Check sheet for the drawn part. Datum: minimum x, y, z corner. Units: mm. A direction names the side the tool comes from. Give positions to 0.01 mm unless a question says otherwise; leave off trailing zeros. Order: outer loops, then holes, each group sorted by start corner. A loop starts at its lowest first (then second) coordinate and runs counter-clockwise, first axis right, second up.
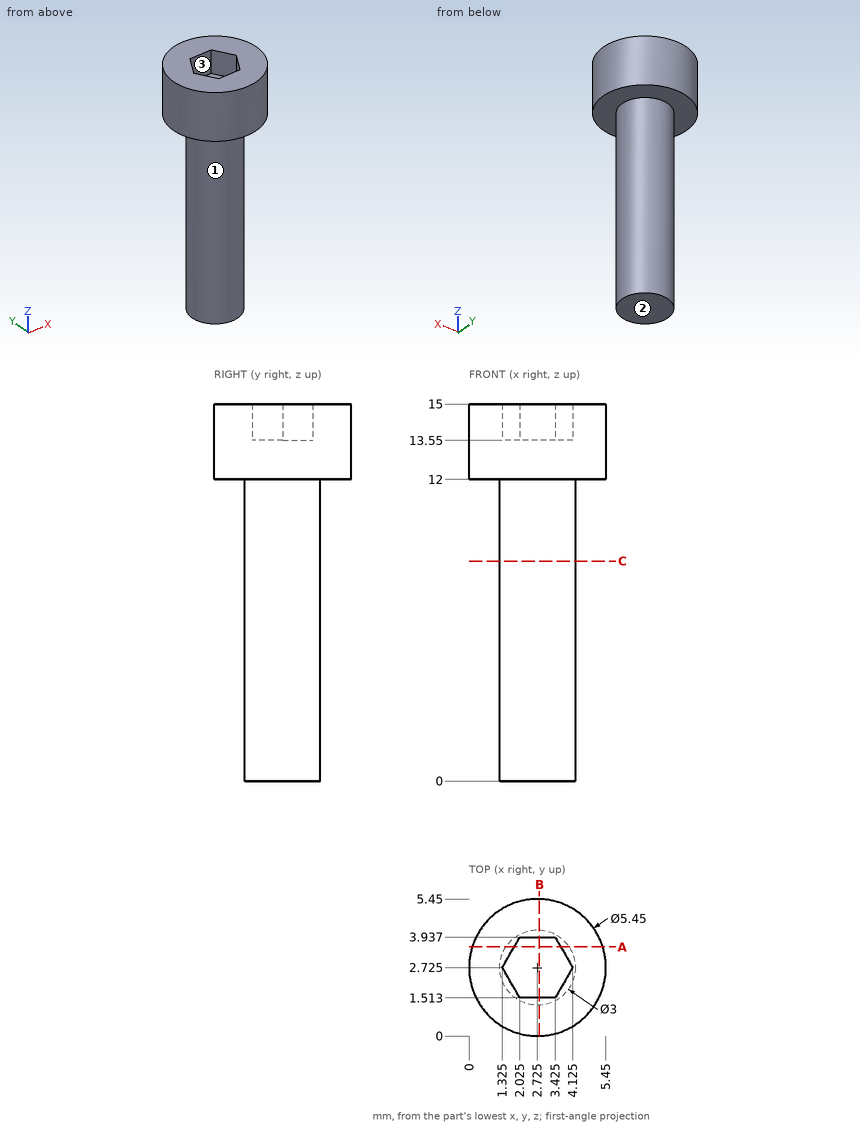
Item 1: Sectioned sample at A-A (y = 3.55). Enter the section's corners in (x, z).
Reported:
outline: (0.13, 12) - (1.47, 12) - (1.47, 0) - (3.98, 0) - (3.98, 12) - (5.32, 12) - (5.32, 15) - (3.65, 15) - (3.65, 13.55) - (1.8, 13.55) - (1.8, 15) - (0.13, 15) - close
Item 2: Sectioned sample at C-C (z = 8.75). Enter the section's corners in (x, y) (1 decimal).
Reported:
outline: circle Ø3 at (2.7, 2.7)
Item 3: Sectioned sample at B-B (x = 2.8). Enter the section's corners in (y, z).
Reported:
outline: (0, 12) - (1.23, 12) - (1.23, 0) - (4.22, 0) - (4.22, 12) - (5.45, 12) - (5.45, 15) - (3.94, 15) - (3.94, 13.55) - (1.51, 13.55) - (1.51, 15) - (0, 15) - close
Item 4: Set-up check for the marked faces 1, 2 and 3: record each of +Z, -Z, +X, -X, +Y, -Y from which the full face is reachable in a straight line by a thin tool's end or side.
Reported:
face 1: -Z
face 2: -Z, +X, -X, +Y, -Y
face 3: +Z
Item 5: Gauge pin test, flat end, axial feed: pin 1 (2 mm diameter, centred on x = 3, z = 4, fed in from +Y) (3 decimals). Record the tip position at first contact, or that the pin passes through.
Reported:
pin 1: stops at y = 4.225
Item 6: Scan lines: L1, parallel to Z at x = 2.65, y = 2.65; L2, parallel to Z at x = 0.85, y = 3.3; L3, parallel to X at y = 4.05, z = 4 (1 decimal). Record each from-to range of solid material in increasing order.
Reported:
L1: z = 0 to 13.55
L2: z = 12 to 15
L3: x = 2 to 3.4
